Part model, mm, in its own coordinate system. Round coordinates to 2 decimals unless told otherwise and drop trailing zeros. Write each loop counter-clockwise with the first axis right and the second up, starting at its lowest first coordinate (ties: lowest second). Pieces come first, ordered by that corner, then holes.
```python
from build123d import *

# Parameters (mm, degrees)
SKETCH1_W           = 1.524
SKETCH1_H           = 19.05
BOSS_EXTRUDE1_DEPTH = 1.524


with BuildPart() as part:
    # Sketch1 → Boss-Extrude1 (new body)
    with BuildSketch(Plane.XY):
        with BuildLine():
            Line((-12.968401667, -214.533069625), (-5.231008599, -219.308220204))
            ThreePointArc((-5.231008599, -219.308220204), (-2.186267033, -216.881335926), (1.524, -215.700600116))
            ThreePointArc((1.524, -215.700600116), (3.189789502, -215.033578347), (4.911266579, -214.527328034))
            ThreePointArc((4.911266579, -214.527328034), (8.56652215, -210.778134694), (8.366250568, -205.545808702))
            ThreePointArc((8.366250568, -205.545808702), (5.494506116, -190.54054727), (13.311403321, -177.414203341))
            ThreePointArc((13.311403321, -177.414203341), (14.109075531, -176.108897248), (14.468404268, -174.621958174))
            ThreePointArc((14.468404268, -174.621958174), (14.169609027, -170.48015642), (14.223154403, -166.327936138))
            ThreePointArc((14.223154403, -166.327936138), (14.204082667, -165.84665661), (14.094500503, -165.377630529))
            ThreePointArc((14.094500503, -165.377630529), (11.21769373, -160.262840376), (6.664633993, -156.56057856))
            ThreePointArc((6.664633993, -156.56057856), (1.308827331, -153.190269752), (-3.738486028, -149.373428868))
            ThreePointArc((-3.738486028, -149.373428868), (-3.917462061, -155.201242728), (-2.164967532, -160.762196757))
            ThreePointArc((-2.164967532, -160.762196757), (-10.348444798, -155.111050325), (-16.602878059, -147.37885654))
            ThreePointArc((-16.602878059, -147.37885654), (-13.34872328, -162.415016966), (-2.254215141, -173.07276217))
            ThreePointArc((-2.254215141, -173.07276217), (-12.048739338, -189.17955679), (-5.548621032, -206.874471292))
            ThreePointArc((-5.548621032, -206.874471292), (-10.108356413, -209.880426072), (-12.968401667, -214.533069625))
        make_face()
        with Locations((0.762, -183.574694423)):
            Rectangle(SKETCH1_W, SKETCH1_H, mode=Mode.SUBTRACT)
    extrude(amount=BOSS_EXTRUDE1_DEPTH)


solid = part.part
```
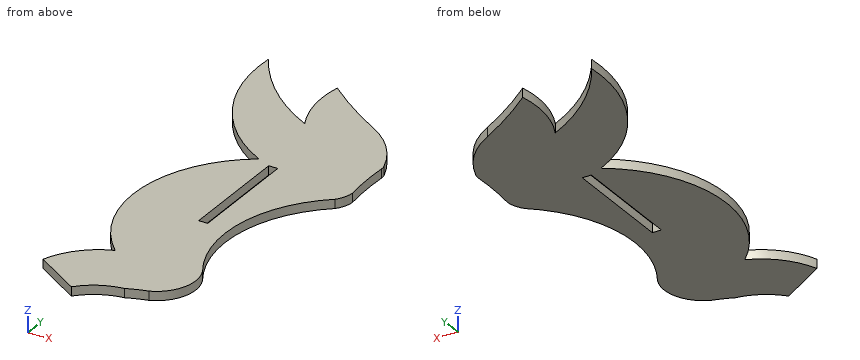
Q1. Drop flat-ended pins along their axis: pin 1 (6 mm diameter, centred on x = -13.5, y = -183.5, fed in from -Z); pin 2 (0.8 mm diameter, centred on x = 1, z = 1, fed in from -Y); pin 3 (0.5 mm diameter, centred on y = -181, z = 0.5, fed in from +X). Give the stop position or say it passes through.
Values follow:
pin 1: stops at z = 0
pin 2: stops at y = -215.86
pin 3: stops at x = 9.95
Q2. Cut at C-C on z = 0.65. Write the cut outline in (x, y) (1 decimal).
Values follow:
outline: (-16.6, -147.4) arc R26.4 ccw to (-2.3, -173.1) arc R21.7 ccw to (-5.5, -206.9) arc R12.6 ccw to (-13, -214.5) - (-5.2, -219.3) arc R10.7 cw to (1.5, -215.7) arc R18.9 cw to (4.9, -214.5) arc R6.6 ccw to (8.4, -205.5) arc R21.5 cw to (13.3, -177.4) arc R4.9 ccw to (14.5, -174.6) arc R48.9 cw to (14.2, -166.3) arc R2.5 ccw to (14.1, -165.4) arc R15.7 ccw to (6.7, -156.6) arc R73.8 cw to (-3.7, -149.4) arc R17.4 ccw to (-2.2, -160.8) arc R34.9 cw to start; hole (0, -193.1) - (1.5, -193.1) - (1.5, -174) - (0, -174) - close
Q3. Cut at B-B on y = -154.5. Write the cut outline in (x, z), plus the area to 3 significant figures.
Values follow:
outline: (-16.23, 0) - (-10.99, 0) - (-10.99, 1.52) - (-16.23, 1.52) - close; (-4, 0) - (3.27, 0) - (3.27, 1.52) - (-4, 1.52) - close
area: 19.1 mm2
Q4. Cut at A-A on x = -3. Write the cut outline in (y, z).
Values follow:
outline: (-217.36, 0) - (-173.58, 0) - (-173.58, 1.52) - (-217.36, 1.52) - close; (-172.68, 0) - (-160.33, 0) - (-160.33, 1.52) - (-172.68, 1.52) - close; (-158.86, 0) - (-149.98, 0) - (-149.98, 1.52) - (-158.86, 1.52) - close
Q5. Wall check: L1, parallel to Y at x = -10.5, z = 1.25; L2, parallel to Y at x = 8.5, z = 0.45; L3, parallel to X at y = -192, z = 0.4. Give the ranges that are in metal, low to high.
Values follow:
L1: y = -216.06 to -210.3, -199.59 to -182.98, -166.54 to -154.97
L2: y = -210.94 to -205.85, -182.77 to -157.72
L3: x = -12.14 to 0, 1.52 to 5.29
Q6. Cut at D-D on y = -182. Write the cut outline in (x, z), plus the area to 3 significant figures.
Values follow:
outline: (-10.06, 0) - (0, 0) - (0, 1.52) - (-10.06, 1.52) - close; (1.52, 0) - (9.01, 0) - (9.01, 1.52) - (1.52, 1.52) - close
area: 26.7 mm2
